Autodesk Inventor part; units mm, degrees
ref_plane "YZ Plane" through (0, 0, 0) normal (1, 0, 0) x (0, 1, 0)
ref_plane "XZ Plane" through (0, 0, 0) normal (0, 1, 0) x (-1, 0, 0)
ref_plane "XY Plane" through (0, 0, 0) normal (0, 0, 1) x (1, 0, 0)
sketch "スケッチ1" plane through (0, 0, 0) normal (0, 0, 1) x (1, 0, 0)
  circle A0 centre (0, 0) radius 20.35
  circle A1 centre (0, 0) radius 8.5
  dimension "d0" = 40.7
  dimension "d1" = 17
extrude "押し出し1" add sketch "スケッチ1" along normal blind 2.5
sketch "スケッチ2" plane through (0, 0, 0) normal (0, 0, -1) x (-1, 0, 0)
  circle A0 centre (0, 15) radius 1.75
  line L0 (0, -28.49) -> (0, 28.49)
  point P0 (0, 0)
  dimension "d4" = 15
  dimension "d5" = 3.5
extrude "押し出し2" cut sketch "スケッチ2" against normal blind 5
pattern_circular "円形状パターン1" count 4 over 360 about axis through (0, 0, -10) along (0, 0, 1) of "押し出し2"
chamfer "面取り1" distance 2 angle 45 1 edges at (-8.5, 0, 2.5)
properties part number "bar2"
Could you check a few things on this model? Use its own coordinates, in mm. Coordinates: 2 decimals unless noted, no trailing zeros. Write each loop counter-clockwise with the first axis right and the second up, starting at its lowest first coordinate (ties: lowest second). Pieces come first, ordered by that corner, then holes. Notation, with made-up numbers: (45.25, 61.25) - (57.25, 61.25) arc R24 cw to (57.25, 93.25) - close; hole circle Ø5 at (-28.75, 29.5). An arc over 180 degrees is marked (long way). Put each result on its own line as item: value. Start each with the question number.
Q1. Thinking about a two-plate mould opening in Y: for faces 1 (the cylindrical face through (-16.735, 0.228, 1.232)), 2 (the cylindrical face through (-4.411, 19.866, 1.232)), 3 (the flat face through (0, -9, 0)), which applies, pulls with the +Y half, pulls with the -Y half, needs draft (parallel to the pull), parting line crosses it, or undercut?
Q2. I want a section at C-C on z = 1.75. Write out the boundary of the cut face in (x, y), plus the area to 3 significant figures.
Q3. Please list where these lines run through material, in increasing order: L1, parallel to Y at x = 0, z = 1.3; L2, parallel to X at y = 1, z = 2.1; L3, parallel to Y at x = -7.5, z = 0.7.
Q4. I want a section at A-A on x = 0. Write out the boundary of the cut face in (y, z), plus the area to 4 significant figures.
Q5. I'm going to push flat-ended pins straight in: P1, Ø13.5, axis at x = 0, y = 0, coming from the -Z side; P2, Ø1, axis at x = -5, y = 7, coming from the +Z side. Where does each tip first touch, or does it pass through?
Q6. I want a section at D-D on y = -15. Write out the boundary of the cut face in (x, z), plus the area to 3 significant figures.
Checks:
1. face 1: undercut
1. face 2: parting line crosses it
1. face 3: needs draft
2. outline: circle Ø40.7 at (0, 0); hole circle Ø3.5 at (-15, 0); hole circle Ø19.5 at (0, 0); hole circle Ø3.5 at (0, -15); hole circle Ø3.5 at (0, 15); hole circle Ø3.5 at (15, 0)
2. area: 964 mm²
3. L1: -20.35 to -16.75, -13.25 to -9.3, 9.3 to 13.25, 16.75 to 20.35
3. L2: -20.33 to -16.44, -13.56 to -10.05, 10.05 to 13.56, 16.44 to 20.33
3. L3: -18.92 to -4.41, 4.41 to 18.92
4. outline: (-20.35, 0) - (-16.75, 0) - (-16.75, 2.5) - (-20.35, 2.5) - close; (-13.25, 0) - (-8.5, 0) - (-8.5, 0.5) - (-10.5, 2.5) - (-13.25, 2.5) - close; (8.5, 0) - (13.25, 0) - (13.25, 2.5) - (10.5, 2.5) - (8.5, 0.5) - close; (16.75, 0) - (20.35, 0) - (20.35, 2.5) - (16.75, 2.5) - close
4. area: 37.75 mm²
5. P1: through
5. P2: z = 1.1
6. outline: (-13.75, 0) - (-1.75, 0) - (-1.75, 2.5) - (-13.75, 2.5) - close; (1.75, 0) - (13.75, 0) - (13.75, 2.5) - (1.75, 2.5) - close
6. area: 60.0 mm²
